from build123d import *

# Parameters (mm, degrees)
SKETCH1_W                 = 305
SKETCH1_H                 = 390
BOSS_EXTRUDE1_DEPTH       = 16
CUT_EXTRUDE4_DEPTH        = 420.061153055
LPATTERN1_COUNT           = 16
LPATTERN1_PITCH           = 22.5
F_8_36_TAPPED_HOLE1_D     = 3.4544
F_8_36_TAPPED_HOLE1_DEPTH = 25
F_8_36_TAPPED_HOLE1_TIP   = 1.037806461
MIRROR1_COPY_1_DEPTH      = 420.061153055
MIRROR1_COPY_2_DEPTH      = 420.061153055
MIRROR1_COPY_3_DEPTH      = 420.061153055
MIRROR1_COPY_4_DEPTH      = 420.061153055
MIRROR1_COPY_5_DEPTH      = 420.061153055
MIRROR1_COPY_6_DEPTH      = 420.061153055
MIRROR1_COPY_7_DEPTH      = 420.061153055
MIRROR1_COPY_8_DEPTH      = 420.061153055
MIRROR1_COPY_9_DEPTH      = 420.061153055
MIRROR1_COPY_10_DEPTH     = 420.061153055
MIRROR1_COPY_11_DEPTH     = 420.061153055
MIRROR1_COPY_12_DEPTH     = 420.061153055
MIRROR1_COPY_13_DEPTH     = 420.061153055
MIRROR1_COPY_14_DEPTH     = 420.061153055
MIRROR1_COPY_15_DEPTH     = 420.061153055


with BuildPart() as part:
    # Sketch1 → Boss-Extrude1 (new body)
    with BuildSketch(Plane.XY):
        with Locations((0, 195)):
            Rectangle(SKETCH1_W, SKETCH1_H)
    extrude(amount=BOSS_EXTRUDE1_DEPTH)

    # Sketch2 → Cut-Extrude4 (cut, through all)
    with BuildSketch(Plane.XY.offset(16)):
        with BuildLine():
            Line((137.5, 32), (132.5, 32))
            ThreePointArc((132.5, 32), (127, 37.5), (132.5, 43))
            Line((132.5, 43), (137.5, 43))
            ThreePointArc((137.5, 43), (143, 37.5), (137.5, 32))
        make_face()
    cut_extrude4 = extrude(amount=-CUT_EXTRUDE4_DEPTH, mode=Mode.SUBTRACT)

    # LPattern1: Cut-Extrude4 ×16
    with Locations(*[(0, i * LPATTERN1_PITCH, 0) for i in range(1, LPATTERN1_COUNT)]):
        add(cut_extrude4, mode=Mode.SUBTRACT)

    # #8-36 Tapped Hole1
    with Locations(Plane(origin=(0, 0, 0), x_dir=(-1, 0, 0), z_dir=(0, -1, 0))):
        with Locations((-125, -8), (0, -8), (125, -8)):
            Hole(F_8_36_TAPPED_HOLE1_D / 2, depth=F_8_36_TAPPED_HOLE1_DEPTH)
            with Locations((0, 0, -(F_8_36_TAPPED_HOLE1_DEPTH + F_8_36_TAPPED_HOLE1_TIP / 2))):  # 118° drill point
                Cone(0, F_8_36_TAPPED_HOLE1_D / 2, F_8_36_TAPPED_HOLE1_TIP, mode=Mode.SUBTRACT)

    # Mirror1: Cut-Extrude4 across plane
    add(cut_extrude4.mirror(Plane(origin=(0, 0, 0), x_dir=(0, 0, 1), z_dir=(1, 0, 0))), mode=Mode.SUBTRACT)

    # Mirror1 copy 1 sketch → Mirror1 copy 1 (cut, through all)
    with BuildSketch(Plane(origin=(0, 22.5, 16), x_dir=(-1, 0, 0), z_dir=(0, 0, 1))):
        with BuildLine():
            Line((137.5, -32), (132.5, -32))
            ThreePointArc((132.5, -32), (127, -37.5), (132.5, -43))
            Line((132.5, -43), (137.5, -43))
            ThreePointArc((137.5, -43), (143, -37.5), (137.5, -32))
        make_face()
    extrude(amount=-MIRROR1_COPY_1_DEPTH, mode=Mode.SUBTRACT)

    # Mirror1 copy 2 sketch → Mirror1 copy 2 (cut, through all)
    with BuildSketch(Plane(origin=(0, 45, 16), x_dir=(-1, 0, 0), z_dir=(0, 0, 1))):
        with BuildLine():
            Line((137.5, -32), (132.5, -32))
            ThreePointArc((132.5, -32), (127, -37.5), (132.5, -43))
            Line((132.5, -43), (137.5, -43))
            ThreePointArc((137.5, -43), (143, -37.5), (137.5, -32))
        make_face()
    extrude(amount=-MIRROR1_COPY_2_DEPTH, mode=Mode.SUBTRACT)

    # Mirror1 copy 3 sketch → Mirror1 copy 3 (cut, through all)
    with BuildSketch(Plane(origin=(0, 67.5, 16), x_dir=(-1, 0, 0), z_dir=(0, 0, 1))):
        with BuildLine():
            Line((137.5, -32), (132.5, -32))
            ThreePointArc((132.5, -32), (127, -37.5), (132.5, -43))
            Line((132.5, -43), (137.5, -43))
            ThreePointArc((137.5, -43), (143, -37.5), (137.5, -32))
        make_face()
    extrude(amount=-MIRROR1_COPY_3_DEPTH, mode=Mode.SUBTRACT)

    # Mirror1 copy 4 sketch → Mirror1 copy 4 (cut, through all)
    with BuildSketch(Plane(origin=(0, 90, 16), x_dir=(-1, 0, 0), z_dir=(0, 0, 1))):
        with BuildLine():
            Line((137.5, -32), (132.5, -32))
            ThreePointArc((132.5, -32), (127, -37.5), (132.5, -43))
            Line((132.5, -43), (137.5, -43))
            ThreePointArc((137.5, -43), (143, -37.5), (137.5, -32))
        make_face()
    extrude(amount=-MIRROR1_COPY_4_DEPTH, mode=Mode.SUBTRACT)

    # Mirror1 copy 5 sketch → Mirror1 copy 5 (cut, through all)
    with BuildSketch(Plane(origin=(0, 112.5, 16), x_dir=(-1, 0, 0), z_dir=(0, 0, 1))):
        with BuildLine():
            Line((137.5, -32), (132.5, -32))
            ThreePointArc((132.5, -32), (127, -37.5), (132.5, -43))
            Line((132.5, -43), (137.5, -43))
            ThreePointArc((137.5, -43), (143, -37.5), (137.5, -32))
        make_face()
    extrude(amount=-MIRROR1_COPY_5_DEPTH, mode=Mode.SUBTRACT)

    # Mirror1 copy 6 sketch → Mirror1 copy 6 (cut, through all)
    with BuildSketch(Plane(origin=(0, 135, 16), x_dir=(-1, 0, 0), z_dir=(0, 0, 1))):
        with BuildLine():
            Line((137.5, -32), (132.5, -32))
            ThreePointArc((132.5, -32), (127, -37.5), (132.5, -43))
            Line((132.5, -43), (137.5, -43))
            ThreePointArc((137.5, -43), (143, -37.5), (137.5, -32))
        make_face()
    extrude(amount=-MIRROR1_COPY_6_DEPTH, mode=Mode.SUBTRACT)

    # Mirror1 copy 7 sketch → Mirror1 copy 7 (cut, through all)
    with BuildSketch(Plane(origin=(0, 157.5, 16), x_dir=(-1, 0, 0), z_dir=(0, 0, 1))):
        with BuildLine():
            Line((137.5, -32), (132.5, -32))
            ThreePointArc((132.5, -32), (127, -37.5), (132.5, -43))
            Line((132.5, -43), (137.5, -43))
            ThreePointArc((137.5, -43), (143, -37.5), (137.5, -32))
        make_face()
    extrude(amount=-MIRROR1_COPY_7_DEPTH, mode=Mode.SUBTRACT)

    # Mirror1 copy 8 sketch → Mirror1 copy 8 (cut, through all)
    with BuildSketch(Plane(origin=(0, 180, 16), x_dir=(-1, 0, 0), z_dir=(0, 0, 1))):
        with BuildLine():
            Line((137.5, -32), (132.5, -32))
            ThreePointArc((132.5, -32), (127, -37.5), (132.5, -43))
            Line((132.5, -43), (137.5, -43))
            ThreePointArc((137.5, -43), (143, -37.5), (137.5, -32))
        make_face()
    extrude(amount=-MIRROR1_COPY_8_DEPTH, mode=Mode.SUBTRACT)

    # Mirror1 copy 9 sketch → Mirror1 copy 9 (cut, through all)
    with BuildSketch(Plane(origin=(0, 202.5, 16), x_dir=(-1, 0, 0), z_dir=(0, 0, 1))):
        with BuildLine():
            Line((137.5, -32), (132.5, -32))
            ThreePointArc((132.5, -32), (127, -37.5), (132.5, -43))
            Line((132.5, -43), (137.5, -43))
            ThreePointArc((137.5, -43), (143, -37.5), (137.5, -32))
        make_face()
    extrude(amount=-MIRROR1_COPY_9_DEPTH, mode=Mode.SUBTRACT)

    # Mirror1 copy 10 sketch → Mirror1 copy 10 (cut, through all)
    with BuildSketch(Plane(origin=(0, 225, 16), x_dir=(-1, 0, 0), z_dir=(0, 0, 1))):
        with BuildLine():
            Line((137.5, -32), (132.5, -32))
            ThreePointArc((132.5, -32), (127, -37.5), (132.5, -43))
            Line((132.5, -43), (137.5, -43))
            ThreePointArc((137.5, -43), (143, -37.5), (137.5, -32))
        make_face()
    extrude(amount=-MIRROR1_COPY_10_DEPTH, mode=Mode.SUBTRACT)

    # Mirror1 copy 11 sketch → Mirror1 copy 11 (cut, through all)
    with BuildSketch(Plane(origin=(0, 247.5, 16), x_dir=(-1, 0, 0), z_dir=(0, 0, 1))):
        with BuildLine():
            Line((137.5, -32), (132.5, -32))
            ThreePointArc((132.5, -32), (127, -37.5), (132.5, -43))
            Line((132.5, -43), (137.5, -43))
            ThreePointArc((137.5, -43), (143, -37.5), (137.5, -32))
        make_face()
    extrude(amount=-MIRROR1_COPY_11_DEPTH, mode=Mode.SUBTRACT)

    # Mirror1 copy 12 sketch → Mirror1 copy 12 (cut, through all)
    with BuildSketch(Plane(origin=(0, 270, 16), x_dir=(-1, 0, 0), z_dir=(0, 0, 1))):
        with BuildLine():
            Line((137.5, -32), (132.5, -32))
            ThreePointArc((132.5, -32), (127, -37.5), (132.5, -43))
            Line((132.5, -43), (137.5, -43))
            ThreePointArc((137.5, -43), (143, -37.5), (137.5, -32))
        make_face()
    extrude(amount=-MIRROR1_COPY_12_DEPTH, mode=Mode.SUBTRACT)

    # Mirror1 copy 13 sketch → Mirror1 copy 13 (cut, through all)
    with BuildSketch(Plane(origin=(0, 292.5, 16), x_dir=(-1, 0, 0), z_dir=(0, 0, 1))):
        with BuildLine():
            Line((137.5, -32), (132.5, -32))
            ThreePointArc((132.5, -32), (127, -37.5), (132.5, -43))
            Line((132.5, -43), (137.5, -43))
            ThreePointArc((137.5, -43), (143, -37.5), (137.5, -32))
        make_face()
    extrude(amount=-MIRROR1_COPY_13_DEPTH, mode=Mode.SUBTRACT)

    # Mirror1 copy 14 sketch → Mirror1 copy 14 (cut, through all)
    with BuildSketch(Plane(origin=(0, 315, 16), x_dir=(-1, 0, 0), z_dir=(0, 0, 1))):
        with BuildLine():
            Line((137.5, -32), (132.5, -32))
            ThreePointArc((132.5, -32), (127, -37.5), (132.5, -43))
            Line((132.5, -43), (137.5, -43))
            ThreePointArc((137.5, -43), (143, -37.5), (137.5, -32))
        make_face()
    extrude(amount=-MIRROR1_COPY_14_DEPTH, mode=Mode.SUBTRACT)

    # Mirror1 copy 15 sketch → Mirror1 copy 15 (cut, through all)
    with BuildSketch(Plane(origin=(0, 337.5, 16), x_dir=(-1, 0, 0), z_dir=(0, 0, 1))):
        with BuildLine():
            Line((137.5, -32), (132.5, -32))
            ThreePointArc((132.5, -32), (127, -37.5), (132.5, -43))
            Line((132.5, -43), (137.5, -43))
            ThreePointArc((137.5, -43), (143, -37.5), (137.5, -32))
        make_face()
    extrude(amount=-MIRROR1_COPY_15_DEPTH, mode=Mode.SUBTRACT)


solid = part.part
Geometry check sheet. Reference: the model listing, model coordinates, mm. Round coordinates to 2 decimals unless told otherwise and drop trailing zeros. Write each loop counter-clockwise with the first axis right and the second up, starting at its lowest first coordinate (ties: lowest second). Pieces come first, ordered by that corner, then holes.
Item 1: Go/stop test with a flat-tipped pin: pin 1 Ø3 at (x, z) = (0, 8) entering from -Y. Record where the tip stops, or that it passes through.
Determined:
pin 1: stops at y = 25.14
Item 2: Section check A-A (y = 105). Record the boundary of the cut face in (x, z), plus the area to 3 significant figures.
Determined:
outline: (-152.5, 0) - (-143, 0) - (-143, 16) - (-152.5, 16) - close; (-127, 0) - (127, 0) - (127, 16) - (-127, 16) - close; (143, 0) - (152.5, 0) - (152.5, 16) - (143, 16) - close
area: 4,370 mm2
Item 3: Material ranges on line 1 along X through (y, z) = (18.5, 8); line 2 along X through (y, z) = (241, 11.25); line 3 along Z through (x, y) = (-125, 17), recorded low to high.
Determined:
line 1: x = -152.5 to -126.73, -123.27 to -1.73, 1.73 to 123.27, 126.73 to 152.5
line 2: x = -152.5 to -142.91, -127.09 to 127.09, 142.91 to 152.5
line 3: z = 0 to 6.27, 9.73 to 16
